Build history of the part. All positions in model axes, mm. A direction names the side the tool comes from. Round coordinates to 2 decimals unless told otherwise and drop trailing zeros. Write each loop counter-clockwise with the first axis right and the second up, starting at its lowest first coordinate (ties: lowest second). Pieces come first, ordered by that corner, then holes. Notation, with made-up numbers: (77.5, -4) - (107.5, -4) arc R22 cw to (107.5, 17) - close; hole circle Ø10 at (44.25, 5.5). An arc over 180 degrees is marked (long way). One line per question, with ' | ' between items.
from build123d import *

# Parameters (mm, degrees)
SKETCH1_R           = 2.5
BOSS_EXTRUDE1_DEPTH = 6
SKETCH3_R           = 1.5
CUT_EXTRUDE2_DEPTH  = 16


with BuildPart() as part:
    # Sketch1 → Boss-Extrude1 (new body)
    with BuildSketch(Plane(origin=(0, 0, 0), x_dir=(1, 0, 0), z_dir=(0, 1, 0))):
        with BuildLine():
            Line((2.193741097, 0.5), (11.989578808, 0.5))
            ThreePointArc((11.989578808, 0.5), (11.782329983, 2.275236289), (11.313708499, 4))
            Line((11.313708499, 4), (3, 4))
            Line((3, 4), (3, 11.618950039))
            ThreePointArc((3, 11.618950039), (-9.637899446, -7.149188365), (11.989578808, -0.5))
            Line((11.989578808, -0.5), (2.193741097, -0.5))
            ThreePointArc((2.193741097, -0.5), (-2.25, 0), (2.193741097, 0.5))
        make_face()
        with Locations(Location((0, -8, 0), (0, 0, 270))):
            Circle(SKETCH1_R, mode=Mode.SUBTRACT)
    extrude(amount=BOSS_EXTRUDE1_DEPTH)

    # Sketch3 → Cut-Extrude2 (cut)
    with BuildSketch(Plane(origin=(0, 0, -4), x_dir=(-1, 0, 0), z_dir=(0, 0, -1))):
        with Locations((-7.16, 3)):
            Circle(SKETCH3_R)
    extrude(amount=-CUT_EXTRUDE2_DEPTH, mode=Mode.SUBTRACT)


solid = part.part
Q1. Saw through at A-A, the plane x = 0. List the corners of the cut face in (y, z), then the cut area to 3 significant figures.
Found:
outline: (0, -12) - (6, -12) - (6, -2.25) - (0, -2.25) - close; (0, 2.25) - (6, 2.25) - (6, 5.5) - (0, 5.5) - close; (0, 10.5) - (6, 10.5) - (6, 12) - (0, 12) - close | area: 87.0 mm^2
Q2. Drill centre lines: L1, parallel to Y at x = 7.16, z = -2; L2, parallel to Z at x = 0.25, y = 5.25; L3, parallel to Z at x = -1.5, y = 5.5. Where is each one in solid material? Low to high. Write a range as from..to.
Found:
L1: 0..1.5, 4.5..6 | L2: -12..-2.24, 2.24..5.51, 10.49..12 | L3: -11.91..-1.68, 1.68..6, 10..11.91
Q3. Pull direction Z, two halves, no side cores. Call faces 4 (the cylindrical face through (5.774, 2.425, -2.274)), 5 (the cylindrical face through (11.787, 2.958, -2.251)), 6 (the cylindrical face through (0.751, 2.958, 10.385)), 7 (the cylindrical face through (-2.25, 2.96, 0.09)): +Z half, -Z half, draft (parallel to the pull), parting line (faces both ways), or undercut.
Found:
face 4: draft | face 5: -Z half | face 6: undercut | face 7: undercut
Q4. Drop flat-ended pins along their axis: pin 1 (1.8 mm diameter, centred on x = 5.5, y = 4, fed in from +Z); pin 2 (3 mm diameter, centred on y = 2.5, z = 8, fed in from -X); pin 3 (1.5 mm diameter, centred on y = 3.5, z = 5.5, fed in from +X); pin 4 (4 mm diameter, centred on x = 0, z = 8, fed in from +Y). Give the stop position or say it passes through.
Found:
pin 1: z = 11.08 | pin 2: x = -10.09 | pin 3: x = 11.02 | pin 4: through
Q5. Saw through at D-D, the plane x = 7.16. List the corners of the cut face in (y, z), then the cut area to 3 significant figures.
Found:
outline: (0, -4) - (1.5, -4) - (1.5, -0.5) - (0, -0.5) - close; (0, 0.5) - (1.5, 0.5) - (1.5, 9.63) - (0, 9.63) - close; (4.5, -4) - (6, -4) - (6, -0.5) - (4.5, -0.5) - close; (4.5, 0.5) - (6, 0.5) - (6, 9.63) - (4.5, 9.63) - close | area: 37.9 mm^2
Q6. Saw through at B-B, the plane y = 2.25. List the corners of the cut face in (x, z), then the cut area to 3 significant figures.
Found:
outline: (2.19, -0.5) arc R2.25 cw (long way) to (2.19, 0.5) - (5.86, 0.5) - (5.86, 10.47) arc R12 ccw (long way) to (3, -11.62) - (3, -4) - (5.86, -4) - (5.86, -0.5) - close; (8.46, -4) - (11.31, -4) arc R12 ccw to (11.99, -0.5) - (8.46, -0.5) - close; (8.46, 0.5) - (11.99, 0.5) arc R12 ccw to (8.46, 8.51) - close; hole circle Ø5 at (0, 8) | area: 332 mm^2
Q7. Saw through at C-C, the plane z = 8. List the corners of the cut face in (x, y).
Found:
outline: (-8.94, 0) - (-2.5, 0) - (-2.5, 6) - (-8.94, 6) - close; (2.5, 0) - (8.94, 0) - (8.94, 6) - (2.5, 6) - close; hole circle Ø3 at (7.16, 3)
Q8. Which spindle directions (+Z, -Z, +X, -X, +Y, -Y) get a long thin tool onto all of the face, cutting with end or side? Do faces 1 (the cylindrical face through (5.774, 2.425, 5.47)), 2 (the flat face through (3, 3, -8)), 3 (the flat face through (5.9, 1.6, -0.5)). Say none if no direction does.
Found:
face 1: +Z, -Z | face 2: -Z, +X, +Y, -Y | face 3: +X, +Y, -Y
